Geometry check sheet. Reference: the model listing, model coordinates, mm. Give positions to 0.01 mm unless a question says otherwise; leave off trailing zeros. Loops run counter-clockwise (first coordinate to the right, second up) from the corner with the lowest first, then second, coordinate; pieces in that order, holes last. Notation, with made-up numbers: (27.25, 16.25) - (38.25, 16.25) arc R8 ccw to (38.25, 25.25) - close; hole circle Ø7 at (39, -25). An arc over 180 degrees is marked (long way). One line per question, with ' | ' between items. Start each with the question number.
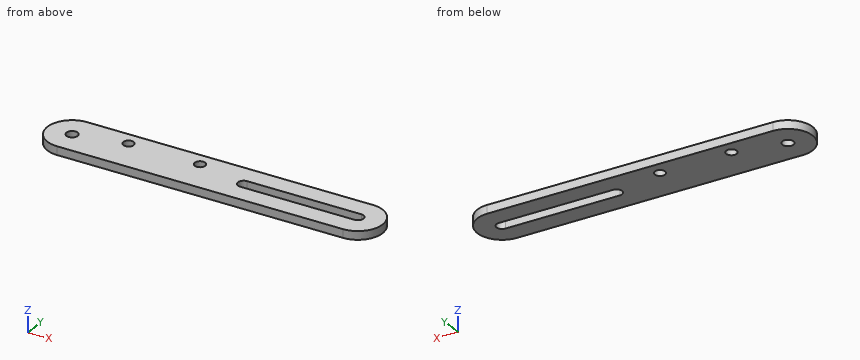
from build123d import *

# Parameters (mm, degrees)
ESQUISSE1_R             = 4
BOSS_EXTRU_1_DEPTH      = 6
ENL_V_MAT_EXTRU_1_REACH = 132.108
ESQUISSE2_R             = 3.75


with BuildPart() as part:
    # Esquisse1 → Boss.-Extru.1 (new body)
    with BuildSketch(Plane.XY):
        with BuildLine():
            Line((-111.286517575, 17.5), (88.713482425, 17.5))
            ThreePointArc((88.713482425, 17.5), (106.213482425, 0), (88.713482425, -17.5))
            Line((88.713482425, -17.5), (-111.286517575, -17.5))
            ThreePointArc((-111.286517575, -17.5), (-128.786517575, 0), (-111.286517575, 17.5))
        make_face()
        with Locations((-111.286517575, 0)):
            Circle(ESQUISSE1_R, mode=Mode.SUBTRACT)
        with BuildLine():
            Line((88.713482425, -4), (8.713482425, -4))
            ThreePointArc((8.713482425, -4), (4.713482425, 0), (8.713482425, 4))
            Line((8.713482425, 4), (88.713482425, 4))
            ThreePointArc((88.713482425, 4), (92.713482425, 0), (88.713482425, -4))
        make_face(mode=Mode.SUBTRACT)
    extrude(amount=BOSS_EXTRU_1_DEPTH)

    # Esquisse2 → Enlèv. mat.-Extru.1 (cut, up to next)
    with BuildSketch(Plane.XY.offset(6), mode=Mode.PRIVATE) as enl_v_mat_extru_1_sk1:
        with Locations((-76.286517575, 7.5)):
            Circle(ESQUISSE2_R)
    enl_v_mat_extru_1_tool1 = extrude(enl_v_mat_extru_1_sk1.sketch, amount=-ENL_V_MAT_EXTRU_1_REACH, mode=Mode.PRIVATE) & part.part
    # Esquisse2 → Enlèv. mat.-Extru.1 (cut, up to next)
    with BuildSketch(Plane.XY.offset(6), mode=Mode.PRIVATE) as enl_v_mat_extru_1_sk2:
        with Locations((-26.286517575, 7.5)):
            Circle(ESQUISSE2_R)
    enl_v_mat_extru_1_tool2 = extrude(enl_v_mat_extru_1_sk2.sketch, amount=-ENL_V_MAT_EXTRU_1_REACH, mode=Mode.PRIVATE) & part.part
    add(enl_v_mat_extru_1_tool1.solids().sort_by_distance((-76.286518, 7.5, 6))[0], mode=Mode.SUBTRACT)
    add(enl_v_mat_extru_1_tool2.solids().sort_by_distance((-26.286518, 7.5, 6))[0], mode=Mode.SUBTRACT)


solid = part.part
(1) Section check A-A, the plane y = 0. Record the boundary of the cut face in (x, z), and give its area (3 significant figures).
(2) Depth check by flat-ended pin: pin 1 Ø1 at (y, z) = (-0.5, 2) entering from -X. Enter the tip coordinate at first touch or a pass-through.
(3) Section check C-C, the plane z = 1.75. Record the boundary of the cut face in (x, y).
(4) Section check D-D, the plane y = -11. Record the boundary of the cut face in (x, z).
(5) Section check B-B, the plane x = -75.5. Record the boundary of the cut face in (y, z), and give its area (3 significant figures).
(6) Material ranges on line 1 (X direction, y = 2.5, z = 2.1); line 2 (Y direction, x = 86, z = 1.4); line 3 (X direction, y = 1, z = 0.45), recorded low to high.
Numbers:
1) outline: (-128.79, 0) - (-115.29, 0) - (-115.29, 6) - (-128.79, 6) - close; (-107.29, 0) - (4.71, 0) - (4.71, 6) - (-107.29, 6) - close; (92.71, 0) - (106.21, 0) - (106.21, 6) - (92.71, 6) - close | area: 834 mm^2
2) pin 1: x = -128.79
3) outline: (-111.29, -17.5) - (88.71, -17.5) arc R17.5 ccw to (88.71, 17.5) - (-111.29, 17.5) arc R17.5 ccw to start; hole circle Ø8 at (-111.29, 0); hole circle Ø7.5 at (-76.29, 7.5); hole circle Ø7.5 at (-26.29, 7.5); hole (8.71, -4) - (88.71, -4) arc R4 ccw to (88.71, 4) - (8.71, 4) arc R4 ccw to start
4) outline: (-124.9, 0) - (102.32, 0) - (102.32, 6) - (-124.9, 6) - close
5) outline: (-17.5, 0) - (3.83, 0) - (3.83, 6) - (-17.5, 6) - close; (11.17, 0) - (17.5, 0) - (17.5, 6) - (11.17, 6) - close | area: 166 mm^2
6) line 1: -128.61 to -114.41, -108.16 to 5.59, 91.84 to 106.03 | line 2: -17.5 to -4, 4 to 17.5 | line 3: -128.76 to -115.16, -107.41 to 4.84, 92.59 to 106.18
